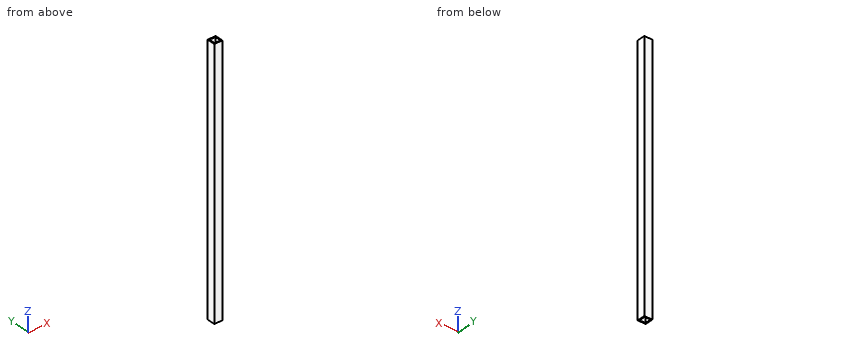
Autodesk Inventor part; units mm, degrees
ref_plane "YZ Plane" through (0, 0, 0) normal (1, 0, 0) x (0, 1, 0)
ref_plane "XZ Plane" through (0, 0, 0) normal (0, 1, 0) x (-1, 0, 0)
ref_plane "XY Plane" through (0, 0, 0) normal (0, 0, 1) x (1, 0, 0)
sketch "Sketch1" plane through (0, 0, 0) normal (0, 0, 1) x (1, 0, 0)
  line L0 (0, 0) -> (25.4, 0)
  line L1 (25.4, 0) -> (25.4, 25.4)
  line L2 (25.4, 25.4) -> (0, 25.4)
  line L3 (0, 25.4) -> (0, 0)
  line L4 (0, 0) -> (0, 3.175)
  line L5 (0, 3.175) -> (3.175, 3.175)
  line L6 (3.175, 3.175) -> (22.225, 3.175)
  line L7 (22.225, 3.175) -> (22.225, 22.225)
  line L8 (22.225, 22.225) -> (3.175, 22.225)
  line L9 (3.175, 22.225) -> (3.175, 3.175)
  dimension "d0" = 25.4
  dimension "d1" = 25.4
  dimension "d2" = 3.175
  dimension "d3" = 3.175
  dimension "d4" = 19.05
  dimension "d5" = 19.05
extrude "Extrusion1" add sketch "Sketch1" along normal blind 812.8
properties part number "32inSquarePipe"
Geometry check sheet. Reference: the model listing, model coordinates, mm. Give positions to 0.01 mm unless a question says otherwise; leave off trailing zeros. Write each loop counter-clockwise with the first axis right and the second up, starting at its lowest first coordinate (ties: lowest second). Pieces come first, ordered by that corner, then holes. Notation, with made-up numbers: (-26.5, -12) - (-12.5, -12) arc R8 ccw to (-12.5, -6) - close; hole circle Ø2 at (4, -35). An arc over 180 degrees is marked (long way). Use a Markdown table: item, result.
Q1. Section check C-C, the plane z = 608.5. Enter the section's corners in (x, y) (3 decimals).
Computed:
| item | result |
|---|---|
| outline | (0, 0) - (25.4, 0) - (25.4, 25.4) - (0, 25.4) - close; hole (3.175, 3.175) - (22.225, 3.175) - (22.225, 22.225) - (3.175, 22.225) - close |
Q2. Thickness scan on L1, parallel to X at y = 12.75, z = 248.5 (3 decimals). Record the ranges inside material, lowest first. Write a range as [from, to].
Computed:
| item | result |
|---|---|
| L1 | x = [0, 3.175], [22.225, 25.4] |
Q3. Go/stop test with a flat-tipped pin: P1, Ø5, axis at y = 17, z = 176, coming from the -X side. Record where the tip stops, or that it passes through.
Computed:
| item | result |
|---|---|
| P1 | stops at x = 0 |
Q4. Section check A-A, the plane x = 14.5. Enter the section's corners in (y, z) (3 decimals).
Computed:
| item | result |
|---|---|
| outline | (0, 0) - (3.175, 0) - (3.175, 812.8) - (0, 812.8) - close; (22.225, 0) - (25.4, 0) - (25.4, 812.8) - (22.225, 812.8) - close |
